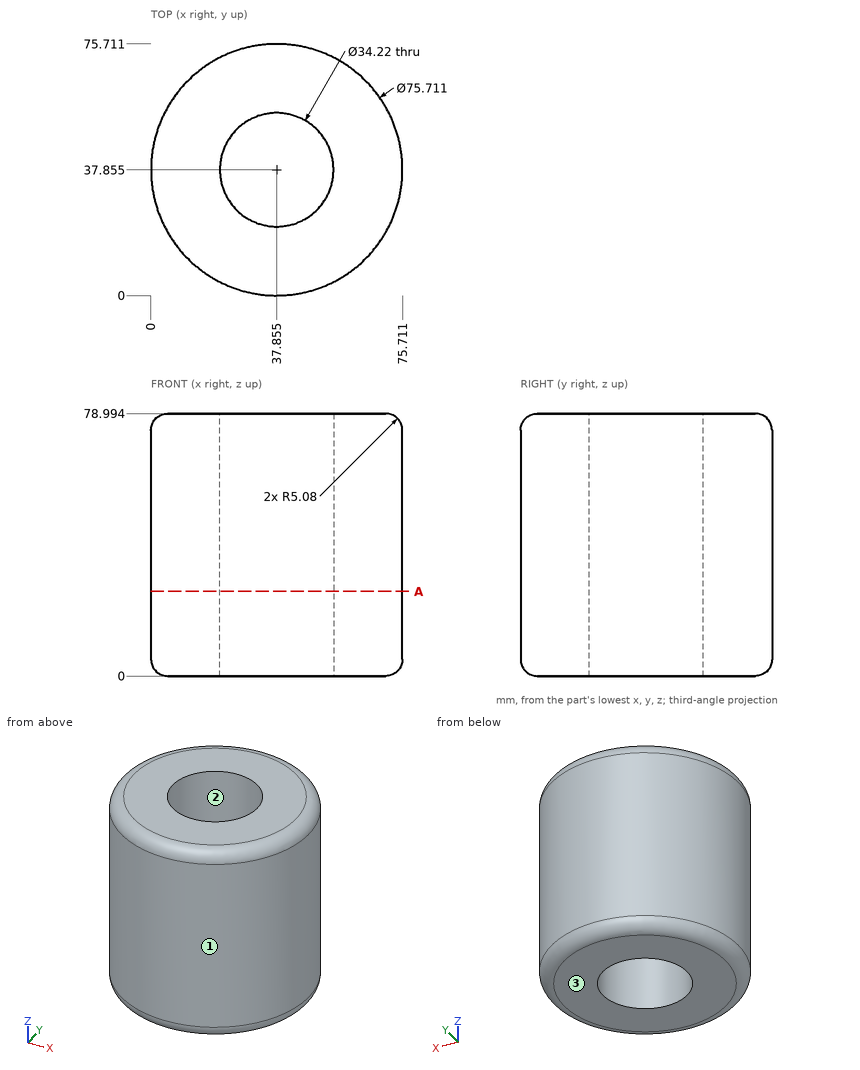
The drawing under review shows one solid part. Ordinate dimensions are in mm from its lowest x, y, z. Give positions to 0.01 mm unless a question says otherwise; leave off trailing zeros. Loops run counter-clockwise (first coordinate to the right, second up) from the corner with the lowest first, then second, coordinate; pieces in that order, holes last. Notation, with made-up numbers: M -27.5,42 L 14.5,42 A10 cw 14.5,49 Z; hole C -35.75,70.25 d4. An arc over 180 degrees is marked long. Return JSON: item names as keys, results as strings. Group by question number.
Item 1: For probe 1 along X at (y, z) = (37, 7); probe 2 along Y at (x, z) = (25.5, 9) (1 decimal); probe 3 along Y at (x, z) = (42, 22.5) (1 decimal), list the stretches that pass through material, from the lowest coordinate up.
Item 2: Insertion check: pin 1 Ø5 at (x, z) = (38, 60.5) entering from -Y; pin 2 Ø8 at (x, z) = (41.5, 11.5) entering from +Y; pin 3 Ø4 at (x, z) = (16, 63) entering from +Y (1 decimal). Each pin has a flat end and moves straight along its axis. Give the tip position at first contact, or say it passes through.
Item 3: We need section A-A (z = 25.5). Give the boundary of the cut face in (x, y) (1 decimal), and give its area (3 significant figures).
Item 4: Mouldability with a two-part tool opening along X and no side actions: class the marked faces 1, 2 and 3 as released by +X, released by -X, zero draft, split by the parting line, or undercut.
Output:
{
 "1": {"probe 1": "x = 0.01 to 20.77, 54.94 to 75.7", "probe 2": "y = 2.1 to 26, 49.7 to 73.6", "probe 3": "y = 0.2 to 21.3, 54.5 to 75.5"},
 "2": {"pin 1": "stops at y = 0", "pin 2": "stops at y = 75.71", "pin 3": "stops at y = 70.1"},
 "3": {"outline": "C 37.9,37.9 d75.7; hole C 37.9,37.9 d34.2", "area": "3,580 mm^2"},
 "4": {"face 1": "split by the parting line", "face 2": "undercut", "face 3": "zero draft"}
}
